The model under review builds one solid part; all positions refer to its coordinate system, in mm. Face numbers are marked on the shaded views. A direction names the side the tool comes from. Coordinates: 2 decimals unless noted, no trailing zeros. Write each loop counter-clockwise with the first axis right and the second up, starting at its lowest first coordinate (ties: lowest second). Pieces come first, ordered by that corner, then holes. Notation, with made-up numbers: (71.5, 55) -> (93.5, 55) arc R32 ccw to (93.5, 91) -> close; hole circle Ø6 at (75.5, -15). An arc over 180 degrees is marked (long way). Put each result on its own line as item: value. Start each with the question number.
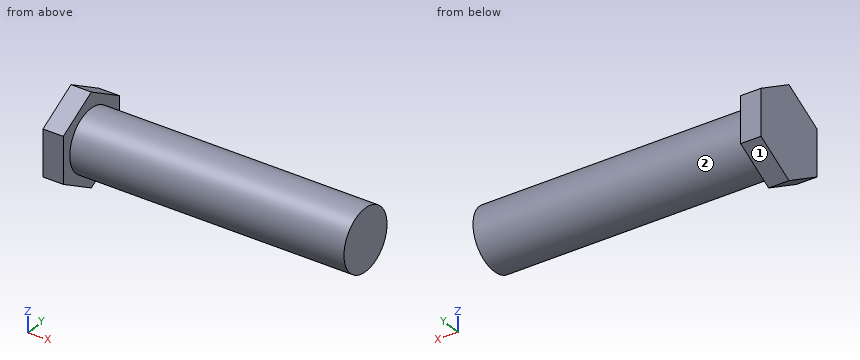
from build123d import *

# Parameters (mm, degrees)
SKETCH1_R           = 29.95
BOSS_EXTRUDE1_DEPTH = 270
BOSS_EXTRUDE2_DEPTH = 20


with BuildPart() as part:
    # Sketch1 → Boss-Extrude1 (new body)
    with BuildSketch(Plane(origin=(0, 0, 0), x_dir=(0, 0, -1), z_dir=(1, 0, 0))):
        Circle(SKETCH1_R)
    extrude(amount=BOSS_EXTRUDE1_DEPTH)

    # Sketch2 → Boss-Extrude2 (add)
    with BuildSketch(Plane.ZY):
        Polygon((45, 0), (22.5, 38.97114317), (-22.5, 38.97114317), (-45, 0), (-22.5, -38.97114317), (22.5, -38.97114317), align=None)
    extrude(amount=BOSS_EXTRUDE2_DEPTH)


solid = part.part
1. Consider section A-A on z = 0. State the section outline as (x, y) points.
2. Tool access review of the marked faces 1 and 2: name each direction out of +Z, -Z, +X, -X, +Y, -Y from which nothing blocks a thin tool from reaching the whole face with its end or side.
3. Consider section B-B on y = 18. State the section outline as (x, z) points.
4. Wall thickness on line 1 (X direction, y = 16, z = -34.5); line 2 (Z direction, x = 52, y = -8.5); line 3 (Z direction, x = 125, y = -11.5): over which ranges is each line inside the solid? List them lowest first. Write a range as from..to.
5. Insertion check: P1, Ø10, axis at x = 27.5, y = 0, coming from the -Z side; P2, Ø5, axis at x = 167, y = 11.5, coming from the -Z side; P3, Ø2, axis at x = 49, z = 7, coming from the +Y side. Each pin has a flat end and moves straight along its axis. Give the tip position at first contact, or say it passes through.
6. Consider section C-C on x = 50. State the section outline as (y, z) points.
7. Consider section D-D on z = -36.5. State the section outline as (x, y) points.
Output values:
1. outline: (-20, -38.97) -> (0, -38.97) -> (0, -29.95) -> (270, -29.95) -> (270, 29.95) -> (0, 29.95) -> (0, 38.97) -> (-20, 38.97) -> close
2. face 1: -Z, +X, -X, +Y
2. face 2: +X
3. outline: (-20, -34.61) -> (0, -34.61) -> (0, -23.94) -> (270, -23.94) -> (270, 23.94) -> (0, 23.94) -> (0, 34.61) -> (-20, 34.61) -> close
4. line 1: x = -20..0
4. line 2: z = -28.72..28.72
4. line 3: z = -27.65..27.65
5. P1: stops at z = -29.95
5. P2: stops at z = -28.57
5. P3: stops at y = 29.34
6. outline: circle Ø59.9 at (0, 0)
7. outline: (-20, -14.72) -> (0, -14.72) -> (0, 14.72) -> (-20, 14.72) -> close
